Check sheet for the modelled part. Datum: model origin and axes. Units: mm. Round coordinates to 2 decimals unless told otherwise and drop trailing zeros. Order: outer loops, then holes, each group sorted by start corner. A loop starts at its lowest first (then second) coordinate and runs counter-clockwise, first axis right, second up. Notation, with made-up numbers: (27.5, -28.5) -> (74.5, -28.5) arc R25 ccw to (74.5, -5.5) -> close; hole circle Ø2 at (2.5, 52). An arc over 180 degrees is marked (long way). Answer in a Markdown table with one row per item.
from build123d import *

# Parameters (mm, degrees)
ESQUISSE1_W             = 48
ESQUISSE1_H             = 46
BOSS_EXTRU_1_DEPTH      = 10
ESQUISSE3_W             = 21
ESQUISSE3_H             = 3.5
ENL_V_MAT_EXTRU_1_DEPTH = 10


with BuildPart() as part:
    # Esquisse1 → Boss.-Extru.1 (new body)
    with BuildSketch(Plane(origin=(0, 0, 0), x_dir=(1, 0, 0), z_dir=(0, 1, 0))):
        with Locations((24, 23)):
            Rectangle(ESQUISSE1_W, ESQUISSE1_H)
    extrude(amount=BOSS_EXTRU_1_DEPTH)

    # Esquisse3 → Enlèv. mat.-Extru.1 (cut)
    with BuildSketch(Plane(origin=(0, 10, 0), x_dir=(1, 0, 0), z_dir=(0, 1, 0))):
        with Locations((36, 4.419258555)):
            Rectangle(ESQUISSE3_W, ESQUISSE3_H)
        with Locations((36, 8.619258555)):
            Rectangle(ESQUISSE3_W, ESQUISSE3_H)
        with Locations((36, 12.819258555)):
            Rectangle(ESQUISSE3_W, ESQUISSE3_H)
        with Locations((36, 17.019258555)):
            Rectangle(ESQUISSE3_W, ESQUISSE3_H)
        with Locations((36, 21.219258555)):
            Rectangle(ESQUISSE3_W, ESQUISSE3_H)
        with Locations((36, 25.419258555)):
            Rectangle(ESQUISSE3_W, ESQUISSE3_H)
        with Locations((36, 29.619258555)):
            Rectangle(ESQUISSE3_W, ESQUISSE3_H)
        with Locations((36, 33.819258555)):
            Rectangle(ESQUISSE3_W, ESQUISSE3_H)
        with Locations((36, 38.019258555)):
            Rectangle(ESQUISSE3_W, ESQUISSE3_H)
        with Locations((36, 42.219258555)):
            Rectangle(ESQUISSE3_W, ESQUISSE3_H)
        with Locations((12, 4.419258555)):
            Rectangle(ESQUISSE3_W, ESQUISSE3_H)
        with Locations((12, 8.619258555)):
            Rectangle(ESQUISSE3_W, ESQUISSE3_H)
        with Locations((12, 12.819258555)):
            Rectangle(ESQUISSE3_W, ESQUISSE3_H)
        with Locations((12, 17.019258555)):
            Rectangle(ESQUISSE3_W, ESQUISSE3_H)
        with Locations((12, 21.219258555)):
            Rectangle(ESQUISSE3_W, ESQUISSE3_H)
        with Locations((12, 25.419258555)):
            Rectangle(ESQUISSE3_W, ESQUISSE3_H)
        with Locations((12, 29.619258555)):
            Rectangle(ESQUISSE3_W, ESQUISSE3_H)
        with Locations((12, 33.819258555)):
            Rectangle(ESQUISSE3_W, ESQUISSE3_H)
        with Locations((12, 38.019258555)):
            Rectangle(ESQUISSE3_W, ESQUISSE3_H)
        with Locations((12, 42.219258555)):
            Rectangle(ESQUISSE3_W, ESQUISSE3_H)
    extrude(amount=-ENL_V_MAT_EXTRU_1_DEPTH, mode=Mode.SUBTRACT)


solid = part.part
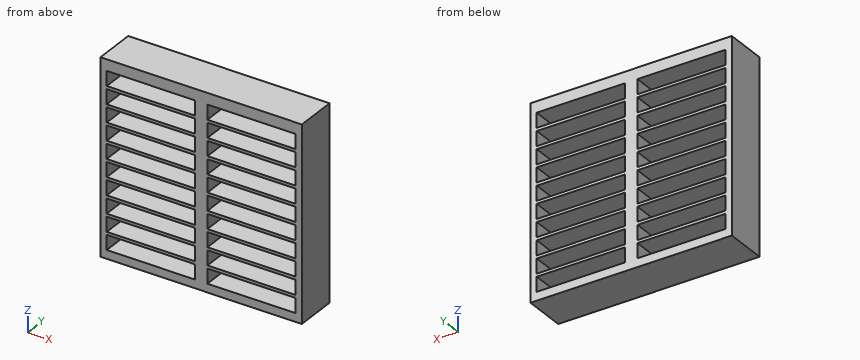
Item 1: Cross-section at A-A (z = -30). Record the boundary of the cut face in (x, y).
Result sheet:
| item | result |
|---|---|
| outline | (0, 0) -> (1.5, 0) -> (1.5, 10) -> (0, 10) -> close; (22.5, 0) -> (25.5, 0) -> (25.5, 10) -> (22.5, 10) -> close; (46.5, 0) -> (48, 0) -> (48, 10) -> (46.5, 10) -> close |
Item 2: Depth check by flat-ended pin: P1, Ø4, axis at x = 10, z = -39.5, coming from the -Y side. Enter the tip coordinate at first touch or a pass-through.
Result sheet:
| item | result |
|---|---|
| P1 | stops at y = 0 |
Item 3: Cross-section at B-B (x = 15). State how many separate pieces and enclosed holes the cut face has, and give its area (3 significant figures).
Result sheet:
| item | result |
|---|---|
| separate pieces | 11 |
| enclosed holes | 0 |
| area | 110 mm^2 |
Item 4: Scan line: line 1 (X direction, y = 6, z = -10). Record every from-to range of solid material in increasing order. Write a range as [from, to].
Result sheet:
| item | result |
|---|---|
| line 1 | x = [0, 1.5], [22.5, 25.5], [46.5, 48] |
